```python
from build123d import *

# Parameters (mm, degrees)
SKETCH_1_W      = 14.6
SKETCH_1_H      = 5.8
EXTRUDE_1_DEPTH = 6


with BuildPart() as part:
    # Эскиз1 → Бобышка-Вытянуть1 (new body)
    with BuildSketch(Plane.XY):
        Polygon((-71.05, -30.4), (71.05, -30.4), (71.05, -17.066666667), (74.45, -17.066666667), (74.45, -6.666666667), (71.05, -6.666666667), (71.05, 6.666666667), (74.45, 6.666666667), (74.45, 17.066666667), (71.05, 17.066666667), (71.05, 30.4), (-71.05, 30.4), (-74.45, 30.4), (-74.45, 16.533333333), (-71.05, 16.533333333), (-71.05, 6.933333333), (-74.45, 6.933333333), (-74.45, -6.933333333), (-71.05, -6.933333333), (-71.05, -16.533333333), (-74.45, -16.533333333), (-74.45, -30.4), align=None)
        with Locations((0, -2.5)):
            Rectangle(SKETCH_1_W, SKETCH_1_H, mode=Mode.SUBTRACT)
        with Locations((-46.1, -2.5)):
            Rectangle(SKETCH_1_W, SKETCH_1_H, mode=Mode.SUBTRACT)
        with Locations((46.1, -2.5)):
            Rectangle(SKETCH_1_W, SKETCH_1_H, mode=Mode.SUBTRACT)
    extrude(amount=EXTRUDE_1_DEPTH)


solid = part.part
```
Check sheet for the modelled part. Datum: model origin and axes. Units: mm. A direction names the side the tool comes from. Round coordinates to 2 decimals unless told otherwise and drop trailing zeros. Loops run counter-clockwise (first coordinate to the right, second up) from the corner with the lowest first, then second, coordinate; pieces in that order, holes last. Notation, with made-up numbers: (-35.5, -21) -> (11.5, -21) arc R25 ccw to (11.5, 13) -> close; hole circle Ø5 at (70, 6.5). An arc over 180 degrees is marked (long way). Answer in a Markdown table with one row per item.
Q1. Thickness scan on L1, parallel to X at y = 11.5, z = 4.65; L2, parallel to X at y = 22, z = 4.05. Record the ranges inside material, lowest first.
Data:
| item | result |
|---|---|
| L1 | x = -71.05 to 74.45 |
| L2 | x = -74.45 to 71.05 |
Q2. Sectioned sample at D-D on y = -24. Enter the section's corners in (x, z).
Data:
| item | result |
|---|---|
| outline | (-74.45, 0) -> (71.05, 0) -> (71.05, 6) -> (-74.45, 6) -> close |
Q3. Release check for a two-part mould opening along X. For faces 4 (the face through (-73, -6.933, 3)), 5 (the face through (-7.3, -3, 3)), 6 (the face through (53.4, -3, 3)), 7 (the face through (74.45, 12, 3)) record: released by +X, released by -X, zero draft, split by the parting line, or undercut.
Data:
| item | result |
|---|---|
| face 4 | zero draft |
| face 5 | undercut |
| face 6 | undercut |
| face 7 | released by +X |
Q4. Set-up check for faces 1 (the face through (0, -5.4, 3)), 2 (the face through (-73, -16.533, 3)), 3 (the face through (73, -17.067, 3)): record each of +Z, -Z, +X, -X, +Y, -Y from which the full face is reachable in a straight line by a thin tool's end or side.
Data:
| item | result |
|---|---|
| face 1 | +Z, -Z |
| face 2 | +Z, -Z, -X |
| face 3 | +Z, -Z, +X, -Y |
Q5. Sectioned sample at B-B on x = -45. Enter the section's corners in (y, z).
Data:
| item | result |
|---|---|
| outline | (-30.4, 0) -> (-5.4, 0) -> (-5.4, 6) -> (-30.4, 6) -> close; (0.4, 0) -> (30.4, 0) -> (30.4, 6) -> (0.4, 6) -> close |
Q6. Sectioned sample at A-A on y = -2.5. Enter the section's corners in (x, z).
Data:
| item | result |
|---|---|
| outline | (-74.45, 0) -> (-53.4, 0) -> (-53.4, 6) -> (-74.45, 6) -> close; (-38.8, 0) -> (-7.3, 0) -> (-7.3, 6) -> (-38.8, 6) -> close; (7.3, 0) -> (38.8, 0) -> (38.8, 6) -> (7.3, 6) -> close; (53.4, 0) -> (71.05, 0) -> (71.05, 6) -> (53.4, 6) -> close |
Q7. Sectioned sample at C-C on z = 5. Give the number of separate pieces and of enclosed holes in the cut face, then the cut area to 3 significant figures.
Data:
| item | result |
|---|---|
| separate pieces | 1 |
| enclosed holes | 3 |
| area | 8,600 mm^2 |
Q8. Go/stop test with flat-tipped pins: P1, Ø1.8, axis at y = 27, z = 3, coming from the +X side; P2, Ø1, axis at x = 72.5, z = 3, coming from the +Y side. Record where each tip stops, or that it passes through.
Data:
| item | result |
|---|---|
| P1 | stops at x = 71.05 |
| P2 | stops at y = 17.07 |
